The model under review builds one solid part; all positions refer to its coordinate system, in mm. Round coordinates to 2 decimals unless told otherwise and drop trailing zeros. Write each loop counter-clockwise with the first axis right and the second up, starting at its lowest first coordinate (ties: lowest second). Pieces come first, ordered by that corner, then holes. Notation, with made-up numbers: M -5.5,82.25 L 37.5,82.25 A14 ccw 37.5,88.25 Z; hole C -16,32.25 d3. An arc over 180 degrees is marked long. One line per item, written item: value. Start each with the question number.
1) For P1, Ø1, axis at y = 246, z = 0.5, coming from the +X side; P2, Ø1.5, axis at y = 278, z = 2, coming from the +X side, all flat-tipped, find the tip position at first contact; note any pin that passes through.
2) Take a section at C-C, the plane x = 287.5. Write out the cut boundary in (y, z).
3) Take a section at B-B, the plane y = 95.5. Write out the cut boundary in (x, z).
4) Take a section at A-A, the plane z = 0.55. Write out the cut boundary in (x, y).
5) Wall thickness on probe 1 along Y at (x, z) = (180, 1.4); probe 2 along X at (y, z) = (332.5, 1.65); probe 3 along X at (y, z) = (8.5, 1.25): over which ranges is each line inside the solid? List them lowest first.
from build123d import *

# Parameters (mm, degrees)
BOSS_EXTRUDE1_DEPTH = 2.5
SKETCH3_R           = 4.5
CUT_EXTRUDE1_DEPTH  = 564.266144908


with BuildPart() as part:
    # Sketch2 → Boss-Extrude1 (new body)
    with BuildSketch(Plane.XY):
        with BuildLine():
            Line((0, 372.5), (0, -372.5))
            Line((0, -372.5), (199.374020374, -372.5))
            ThreePointArc((199.374020374, -372.5), (422.5, 0), (199.374020374, 372.5))
            Line((199.374020374, 372.5), (0, 372.5))
        make_face()
    extrude(amount=BOSS_EXTRUDE1_DEPTH)

    # Sketch3 → Cut-Extrude1 (cut, symmetric)
    with BuildSketch(Plane(origin=(0, 0, 0), x_dir=(-1, 0, 0), z_dir=(0, 0, -1))):
        with Locations((-180, 357.5)):
            Circle(SKETCH3_R)
        with Locations((-180, 332.5)):
            Circle(SKETCH3_R)
    cut_extrude1 = extrude(amount=CUT_EXTRUDE1_DEPTH, both=True, mode=Mode.SUBTRACT)

    # Mirror1: Cut-Extrude1 across plane
    add(cut_extrude1.mirror(Plane.ZX), mode=Mode.SUBTRACT)


solid = part.part
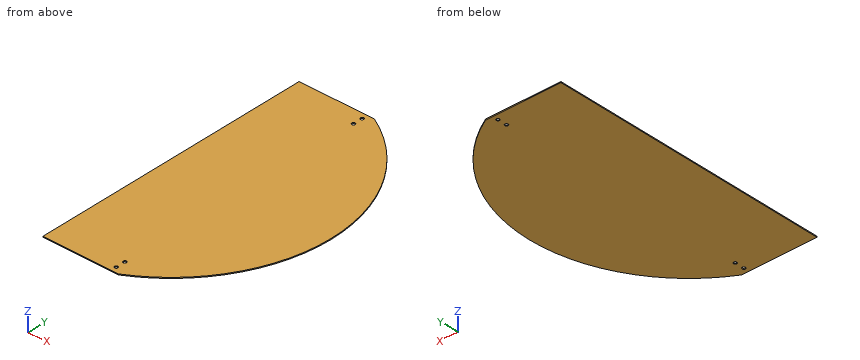
Checked values:
1. P1: stops at x = 343.85
1. P2: stops at x = 318.81
2. outline: M -309.6,0 L 309.6,0 L 309.6,2.5 L -309.6,2.5 Z
3. outline: M 0,0 L 411.57,0 L 411.57,2.5 L 0,2.5 Z
4. outline: M 0,-372.5 L 199.37,-372.5 A422.5 ccw 199.37,372.5 L 0,372.5 Z; hole C 180,-357.5 d9; hole C 180,-332.5 d9; hole C 180,332.5 d9; hole C 180,357.5 d9
5. probe 1: y = -372.5 to -362, -353 to -337, -328 to 328, 337 to 353, 362 to 372.5
5. probe 2: x = 0 to 175.5, 184.5 to 260.67
5. probe 3: x = 0 to 422.41
